Autodesk Inventor part; units mm, degrees
ref_plane "YZ Plane" through (0, 0, 0) normal (1, 0, 0) x (0, 1, 0)
ref_plane "XZ Plane" through (0, 0, 0) normal (0, 1, 0) x (-1, 0, 0)
ref_plane "XY Plane" through (0, 0, 0) normal (0, 0, 1) x (1, 0, 0)
sketch "Sketch1" plane through (0, 0, 0) normal (0, 1, 0) x (-1, 0, 0)
  line L0 (0, 0) -> (-70, 0)
  line L1 (-70, 0) -> (-70, -90)
  line L2 (-70, -90) -> (0, -90)
  line L3 (0, -90) -> (0, 0)
  dimension "d0" = 70
  dimension "d1" = 90
extrude "Extrusion1" add sketch "Sketch1" along normal blind 2
sketch "Sketch2" plane through (70, 0, 0) normal (1, 0, 0) x (0, 0, -1)
  line L0 (0, 2) -> (90, 2)
  line L1 (0, 2) -> (90, 2)
  line L2 (90, 2) -> (90, -38)
  line L3 (90, -38) -> (0, -38)
  line L4 (0, -38) -> (0, 2)
  point P0 (0, 0)
  dimension "d4" = 90
  dimension "d5" = 40
extrude "Extrusion2" add sketch "Sketch2" along normal blind 2
sketch "Sketch3" plane through (0, 0, -90) normal (-1, 0, 0) x (0, 0, 1)
  line L0 (0, 2) -> (90, 2)
  line L1 (90, -38) -> (0, -38)
  line L2 (0, 2) -> (90, 2)
  line L3 (90, 2) -> (90, -38)
  line L4 (90, -38) -> (0, -38)
  line L5 (0, -38) -> (0, 2)
  point P0 (90, 0)
extrude "Extrusion3" add sketch "Sketch3" along normal blind 2
sketch "Sketch4" plane through (70, -38, -90) normal (0, -1, 0) x (1, 0, 0)
  line L0 (0, 90) -> (0, 0)
  line L1 (0, 0) -> (15, 0)
  line L2 (15, 0) -> (15, 90)
  line L3 (15, 90) -> (0, 90)
  line L4 (0, 90) -> (0, 0)
  line L5 (-70, 0) -> (-70, 90)
  line L6 (-70, 0) -> (-85, 0)
  line L7 (-85, 0) -> (-85, 90)
  line L8 (-85, 90) -> (-70, 90)
  line L9 (-70, 90) -> (-70, 0)
  dimension "d10" = 15
  dimension "d11" = 15
extrude "Extrusion4" add sketch "Sketch4" along normal blind 2
sketch "Sketch5" plane through (72, 0, 0) normal (1, 0, 0) x (0, 0, -1)
  arc A0 (16.399, -7.5) -> (16.399, -12.5) centre (11.5, -10) ccw
  line L0 (0, 2) -> (0, -38)
  line L1 (0, 0) -> (90, 0)
  arc A1 (17.5, -12.5) -> (17.5, -7.5) centre (17.5, -10) ccw
  line L2 (17.5, -7.5) -> (16.399, -7.5)
  line L3 (17.5, -12.5) -> (16.399, -12.5)
  dimension "d14" = 11
  dimension "d15" = 11.5
  dimension "d18" = 5
extrude "Extrusion5" cut sketch "Sketch5" against normal blind 95
properties part number "wc" material "Wood (Birch)"
Check sheet for the modelled part. Datum: model origin and axes. Units: mm. A direction names the side the tool comes from. Give positions to 0.01 mm unless a question says otherwise; leave off trailing zeros. Order: outer loops, then holes, each group sorted by start corner. A loop starts at its lowest first (then second) coordinate and runs counter-clockwise, first axis right, second up. Notation, with made-up numbers: (1.25, 62) - (47.25, 62) arc R23 ccw to (47.25, 97) - close; hole circle Ø6 at (21, -18). An arc over 180 degrees is marked (long way). Answer as CSV lines item,"result".
1. Scan lines: probe 1 along X at (y, z) = (-35, -70.5); probe 2 along Y at (x, z) = (70.75, -11.5); probe 3 along Y at (x, z) = (60.5, -9). Record each from-to range of solid material in increasing order. Write a range as from..to.
Result sheet:
probe 1,"-2..0, 70..72"
probe 2,"-40..-15.5, -4.5..2"
probe 3,"0..2"
2. Go/stop test with flat-tipped pins: P1, Ø20, axis at y = -18, z = -53, coming from the -X side; P2, Ø4, axis at x = 14.5, z = -10, coming from the -Y side; P3, Ø4, axis at y = -34, z = -79.5, coming from the +X side; P4, Ø12, axis at x = 6.5, y = -3.5, coming from the +Z side. Record where each tip stops, or that it passes through.
Result sheet:
P1,"x = -2"
P2,"y = 0"
P3,"x = 72"
P4,"z = 0"
3. Section check C-C (y = -21.5). Record the boundary of the cut face in (x, z), then the cut area to 3 significant figures.
Result sheet:
outline,"(-2, -90) - (0, -90) - (0, 0) - (-2, 0) - close; (70, -90) - (72, -90) - (72, 0) - (70, 0) - close"
area,"360 mm²"
4. Mould release check, pull along Z, two halves, no side actions. Record for faces 1 (the face through (17, 1, -90)), 2 (the face through (17, 1, 0)), 3 (the face through (-8, -40, -44)), 4 (the face through (-1, -10, -20)): released by +Z, released by -Z, zero draft, split by the parting line, or undercut.
Result sheet:
face 1,"released by -Z"
face 2,"released by +Z"
face 3,"zero draft"
face 4,"undercut"
5. Section check D-D (z = -32.5). Record the boundary of the cut face in (x, y), then the cut area to 3 significant figures.
Result sheet:
outline,"(-15, -40) - (0, -40) - (0, 0) - (70, 0) - (70, -40) - (85, -40) - (85, -38) - (72, -38) - (72, 2) - (-2, 2) - (-2, -38) - (-15, -38) - close"
area,"360 mm²"
6. Tool access check on faces 5 (the face through (72, -18, -44)), 6 (the face through (71, -10, -20)), 7 (the face through (-9, -38, -44)), 8 (the face through (77, -40, -44)), 9 (the face through (0, -20, -46)). Record the directions out of +Z, -Z, +X, -X, +Y, -Y that give a thin tool (end or side, any length) a straight path to the whole face; none if there is none.
Result sheet:
face 5,"+Z, -Z, +X, +Y"
face 6,"+X, -X"
face 7,"+Z, -Z, -X, +Y"
face 8,"+Z, -Z, +X, -X, -Y"
face 9,"+Z, -Z, -Y"
7. Section check B-B (y = -10). Record the boundary of the cut face in (x, z), then the cut area to 3 significant figures.
Result sheet:
outline,"(-2, -90) - (0, -90) - (0, -20) - (-2, -20) - close; (-2, -6) - (0, -6) - (0, 0) - (-2, 0) - close; (70, -90) - (72, -90) - (72, -20) - (70, -20) - close; (70, -6) - (72, -6) - (72, 0) - (70, 0) - close"
area,"304 mm²"
8. Section check A-A (z = -11.5). Record the boundary of the cut face in (x, y), then the cut area to 3 significant figures.
Result sheet:
outline,"(-15, -40) - (0, -40) - (0, -15.5) - (-2, -15.5) - (-2, -38) - (-15, -38) - close; (-2, -4.5) - (0, -4.5) - (0, 0) - (70, 0) - (70, -4.5) - (72, -4.5) - (72, 2) - (-2, 2) - close; (70, -40) - (85, -40) - (85, -38) - (72, -38) - (72, -15.5) - (70, -15.5) - close"
area,"316 mm²"
